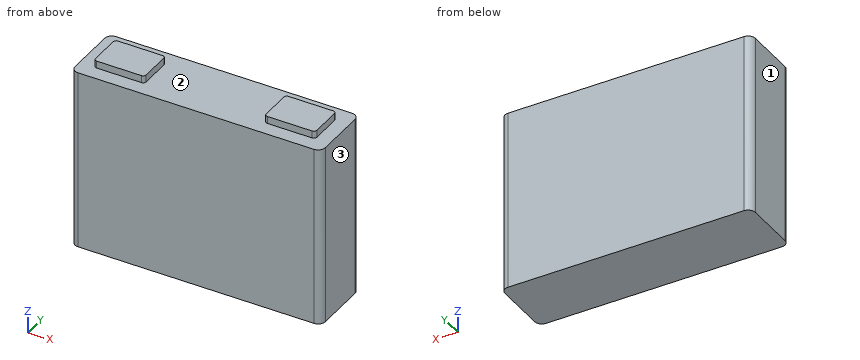
from build123d import *

# Parameters (mm, degrees)
F0_W     = 173
F0_H     = 125
F1_DEPTH = 45
F2_R     = 5
F3_R     = 5
F5_DEPTH = 5


# Not quite as in the source:
# - a pattern or mirror of a feature is missing from the dataset's text; its kind, count and spacing are read off the source's solid


with BuildPart() as f1:
    # F0 (on Front) → F1 (new body)
    with BuildSketch(Plane.XZ):
        with Locations((-86.5, 62.5)):
            Rectangle(F0_W, F0_H)
    extrude(amount=-F1_DEPTH)

    # F2
    f2_edges = [f1.edges().sort_by_distance(p)[0] for p in [
        (0, 0, 62.5),
    ]]
    fillet(f2_edges, radius=F2_R)

    # F3
    f3_edges = [f1.edges().sort_by_distance(p)[0] for p in [
        (0, 45, 62.5),
        (-173, 45, 62.5),
        (-173, 0, 62.5),
    ]]
    fillet(f3_edges, radius=F3_R)

    # F4 (on face) → F5 (join)
    with BuildSketch(Plane.XY.offset(125)):
        with BuildLine():
            Line((-130, 35), (-161, 35))
            ThreePointArc((-161, 35), (-162.4142135624, 34.4142135624), (-163, 33))
            Line((-163, 33), (-163, 12))
            ThreePointArc((-163, 12), (-162.4142135624, 10.5857864376), (-161, 10))
            Line((-161, 10), (-130, 10))
            ThreePointArc((-130, 10), (-128.5857864376, 10.5857864376), (-128, 12))
            Line((-128, 12), (-128, 33))
            ThreePointArc((-128, 33), (-128.5857864376, 34.4142135624), (-130, 35))
        make_face()
    f5 = extrude(amount=F5_DEPTH)

    # F5_copies: F5 across plane
    add(f5.mirror(Plane(origin=(-86.5, 0, 0), x_dir=(0, 0, 1), z_dir=(1, 0, 0))))


solid = f1.part
Can you work these out from the model? Positions are in its coordinate system, mm. Face numbers are marked on the shaded views. Coordinates: 2 decimals unless noted, no trailing zeros. Write each loop counter-clockwise with the first axis right and the second up, starting at its lowest first coordinate (ties: lowest second). Pieces come first, ordered by that corner, then holes.
Q1. Imagine slicing it at A-A, the plane y = 28. List the corners of the cut face in (x, z) for me.
Results found:
outline: (-173, 0) - (0, 0) - (0, 125) - (-10, 125) - (-10, 130) - (-45, 130) - (-45, 125) - (-128, 125) - (-128, 130) - (-163, 130) - (-163, 125) - (-173, 125) - close
Q2. If we mould it in two halves opening along X, with no side actions, what happens to the marked faces 1, 2 and 3? For each: +X half, -X half, draft (parallel to the pull), parting line (faces both ways), or undercut.
Results found:
face 1: -X half
face 2: undercut
face 3: +X half
Q3. Please list where these lines run through material, in increasing order: L1, parallel to Z at x = -131.5, y = 5.5; L2, parallel to X at y = 43, z = 86.5; L3, parallel to X at y = 41, z = 53.
Results found:
L1: z = 0 to 125
L2: x = -172 to -1
L3: x = -172.9 to -0.1
Q4. Imagine slicing it at B-B, the plane x = -40.5. List the corners of the cut face in (y, z) for me.
Results found:
outline: (0, 0) - (45, 0) - (45, 125) - (35, 125) - (35, 130) - (10, 130) - (10, 125) - (0, 125) - close
Q5. For P1, Ø1.5, axis at x = -23.5, z = 128.5, coming from the +Y side; P2, Ø1.5, axis at x = -138.5, z = 128.5, coming from the -Y side; P3, Ø2.5, axis at y = 17.5, z = 128.5, coming from the -X side, each with a flat end and sliding along its axis, tell me the tip position at first contact or that it passes through.
Results found:
P1: stops at y = 35
P2: stops at y = 10
P3: stops at x = -163
Q6. Imagine slicing it at C-C, the plane x = -125.5. List the corners of the cut face in (y, z) for me.
Results found:
outline: (0, 0) - (45, 0) - (45, 125) - (0, 125) - close
